```python
from build123d import *

# Parameters (mm, degrees)
F0_W     = 76.2
F0_H     = 127
F1_DEPTH = 3.175
F2_W     = 38.1
F2_H     = 6.35
F3_DEPTH = 3.175
F4_W     = 1.778
F4_H     = 12.7
F5_DEPTH = 12.7
F6_R     = 6.35
F7_R     = 6.34999
F8_R     = 4.445
F9_DEPTH = 25.4


# Not quite as in the source:
# - a fillet or chamfer is up to 0.001 mm smaller than in the source, because OpenCascade refuses the exact size


with BuildPart() as f1:
    # F0 (on Front) → F1 (new body)
    with BuildSketch(Plane.XZ):
        with Locations((1.208204776, 15.0653144508)):
            Rectangle(F0_W, F0_H)
    extrude(amount=F1_DEPTH)

    # F2 (on face) → F3 (cut)
    with BuildSketch(Plane.XZ.offset(3.175)):
        with Locations((1.208204776, 60.1503144508)):
            Rectangle(F2_W, F2_H)
        with Locations((1.208204776, 48.7203144508)):
            Rectangle(F2_W, F2_H)
        with Locations((1.208204776, 37.2903144508)):
            Rectangle(F2_W, F2_H)
    extrude(amount=-F3_DEPTH, mode=Mode.SUBTRACT)

    # F4 (on face) → F5 (join)
    with BuildSketch(Plane.XZ.offset(3.175)):
        with Locations((37.657204776, 6.35)):
            Rectangle(F4_W, F4_H)
    extrude(amount=F5_DEPTH)

    # F6
    f6_edges = [f1.edges().sort_by_distance(p)[0] for p in [
        (37.657205, -15.875, 12.7),
    ]]
    fillet(f6_edges, radius=F6_R)

    # F7 (radius 6.35 in the source; OpenCascade refuses exactly that, so slightly less here)
    f7_edges = [f1.edges().sort_by_distance(p)[0] for p in [
        (37.657205, -15.875, 0),
    ]]
    fillet(f7_edges, radius=F7_R)

    # F8 (on face) → F9 (cut)
    with BuildSketch(Plane(origin=(36.768204776, 0, 0), x_dir=(0, -1, 0), z_dir=(-1, 0, 0))):
        with Locations((9.525, 6.35)):
            Circle(F8_R)
    extrude(amount=-F9_DEPTH, mode=Mode.SUBTRACT)


solid = f1.part
```
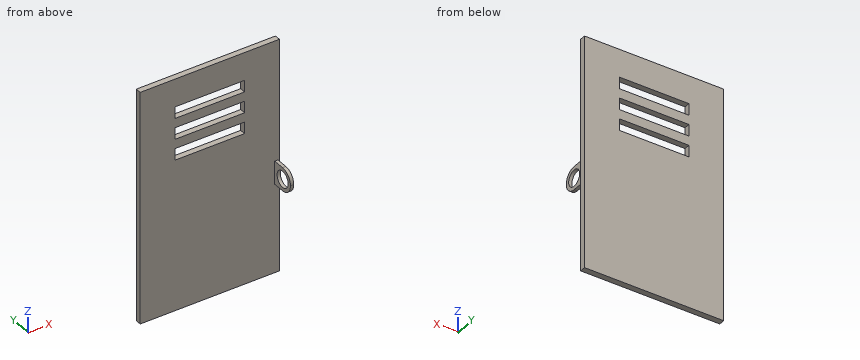
Geometry check sheet. Reference: the model listing, model coordinates, mm. Give positions to 0.01 mm unless a question says otherwise; leave off trailing zeros. Loops run counter-clockwise (first coordinate to the right, second up) from the corner with the lowest first, then second, coordinate; pieces in that order, holes last. Notation, with made-up numbers: M 14.5,80.5 L 18.5,80.5 A30 cw 18.5,110.5 Z; hole C -32.75,3.5 d3. An arc over 180 degrees is marked long. Write item = value, one per line. Start each with the question number.
1. Section check A-A, the plane x = -13. Enter the section's corners in (y, z) (3 decimals).
2. Thickness scan on probe 1 along X at (y, z) = (-2.5, 48); probe 2 along Y at (x, z) = (28, 23) (3 decimals); probe 3 along Y at (x, z) = (37, 6). Record the ranges inside material, lowest first.
3. Section check B-B, the plane z = -26.5. Enter the section's corners in (x, y) (3 decimals), plus the area to 3 significant figures.
4. Section check C-C, the plane x = 26. Enter the section's corners in (y, z) (3 decimals).
5. Go/stop test with flat-tipped pins: P1, Ø2, axis at x = 38, y = -6, coming from the +Z side; P2, Ø4, axis at x = -17, z = 60.5, coming from the -Y side (3 decimals); P3, Ø0.9, axis at x = 37.5, y = -6, coming from the -Z side. Record where each tip stops, or that it passes through.
Values follow:
q1.outline = M -3.175,-48.435 L 0,-48.435 L 0,34.115 L -3.175,34.115 Z; M -3.175,40.465 L 0,40.465 L 0,45.545 L -3.175,45.545 Z; M -3.175,51.895 L 0,51.895 L 0,56.975 L -3.175,56.975 Z; M -3.175,63.325 L 0,63.325 L 0,78.565 L -3.175,78.565 Z
q2.probe_1 = -36.89 to -17.84, 20.26 to 39.31
q2.probe_2 = -3.175 to 0
q2.probe_3 = -15.87 to -13.96, -5.09 to 0
q3.outline = M -36.892,-3.175 L 39.308,-3.175 L 39.308,0 L -36.892,0 Z
q3.area = 242 mm^2
q4.outline = M -3.175,-48.435 L 0,-48.435 L 0,78.565 L -3.175,78.565 Z
q5.P1 = 12.7
q5.P2 = -3.175
q5.P3 = 0
